Design review of the part built by this model. Coordinates are the model's own, in mm. A direction names the side the tool comes from. Give positions to 0.01 mm unless a question says otherwise; leave off trailing zeros. Write each loop counter-clockwise with the first axis right and the second up, starting at its lowest first coordinate (ties: lowest second). Pieces come first, ordered by that corner, then holes. Notation, with made-up numbers: (82.25, 9.5) -> (93.25, 9.5) arc R6 ccw to (93.25, 17.5) -> close; hole circle Ø3 at (8, 35.25). An arc over 180 degrees is marked (long way). Use CSV: the item, a comma, the result in double quotes.
```python
from build123d import *

# Parameters (mm, degrees)
BOSS_EXTRUDE2_DEPTH      = 3
BOSS_EXTRUDE2_DEPTH_BACK = 3
SKETCH2_W                = 50
SKETCH2_H                = 22
SKETCH2_W_2              = 22
SKETCH2_H_2              = 4
BOSS_EXTRUDE3_DEPTH      = 20
BOSS_EXTRUDE3_DEPTH_BACK = 20
SKETCH2_3_W              = 50
SKETCH2_3_H              = 3


with BuildPart() as part:
    # Sketch2 → Boss-Extrude2 (new, two sides: drawn at the far end of the back side and taken through both)
    with BuildSketch(Plane(origin=(0, 0, 0), x_dir=(0, 0, -1), z_dir=(1, 0, 0)).offset(-BOSS_EXTRUDE2_DEPTH_BACK)):
        with Locations((0, -1.5)):
            Rectangle(SKETCH2_W, SKETCH2_H)
        with Locations((0, -7.5)):
            Rectangle(SKETCH2_W_2, SKETCH2_H_2, mode=Mode.SUBTRACT)
    extrude(amount=BOSS_EXTRUDE2_DEPTH + BOSS_EXTRUDE2_DEPTH_BACK)

    # Sketch2<3> → Boss-Extrude3 (add, two sides: drawn at the far end of the back side and taken through both)
    with BuildSketch(Plane(origin=(0, 0, 0), x_dir=(0, 0, -1), z_dir=(1, 0, 0)).offset(-BOSS_EXTRUDE3_DEPTH_BACK)):
        with Locations((0, 11)):
            Rectangle(SKETCH2_3_W, SKETCH2_3_H)
    extrude(amount=BOSS_EXTRUDE3_DEPTH + BOSS_EXTRUDE3_DEPTH_BACK)


solid = part.part
```
(1) Tool access review of faces 5 (the face through (3, -1, 0)), 6 (the face through (0, -5.5, 0)), 7 (the face through (0, 12.5, 0)): name each direction out of +Z, -Z, +X, -X, +Y, -Y from which nothing blocks a thin tool from reaching the whole face with its end or side.
Established:
face 5,"+Z, -Z, +X, -Y"
face 6,"+X, -X"
face 7,"+Z, -Z, +X, -X, +Y"
(2) Take a section at D-D (x = 8). Write out the cut boundary in (y, z).
Established:
outline,"(9.5, -25) -> (12.5, -25) -> (12.5, 25) -> (9.5, 25) -> close"
(3) Take a section at B-B (x = -0.5). Write out the cut boundary in (y, z).
Established:
outline,"(-12.5, -25) -> (12.5, -25) -> (12.5, 25) -> (-12.5, 25) -> close; hole (-9.5, -11) -> (-5.5, -11) -> (-5.5, 11) -> (-9.5, 11) -> close"
(4) Clearance check with flat-ended pins moving along their axes: pin 1 (13.5 mm diameter, centred on x = -12.5, z = -6.5, fed in from -Y); pin 2 (13.5 mm diameter, centred on x = 8.5, z = -12, fed in from -Y); pin 3 (6 mm diameter, centred on y = -0.5, z = 9, fed in from +X); pin 4 (5 mm diameter, centred on y = -2.5, z = -8.5, fed in from -X). State where each tip first meets the part, or that it passes through.
Established:
pin 1,"stops at y = 9.5"
pin 2,"stops at y = -12.5"
pin 3,"stops at x = 3"
pin 4,"stops at x = -3"
(5) Take a section at C-C (z = 16). Write out the cut boundary in (x, y).
Established:
outline,"(-20, 9.5) -> (-3, 9.5) -> (-3, -12.5) -> (3, -12.5) -> (3, 9.5) -> (20, 9.5) -> (20, 12.5) -> (-20, 12.5) -> close"
(6) For line 1 along Y through (x, z) = (-17, -21.5); line 2 along X through (y, z) = (-1.5, 9); line 3 along Z through (x, y) = (0, -8), list the stretches that pass through material, from the lowest coordinate up. Write a range as [from, to].
Established:
line 1,"y = [9.5, 12.5]"
line 2,"x = [-3, 3]"
line 3,"z = [-25, -11], [11, 25]"
(7) Take a section at A-A (z = -1). Write out the cut boundary in (x, y), then the cut area to 3 significant figures.
Established:
outline,"(-20, 9.5) -> (-3, 9.5) -> (-3, -5.5) -> (3, -5.5) -> (3, 9.5) -> (20, 9.5) -> (20, 12.5) -> (-20, 12.5) -> close; (-3, -12.5) -> (3, -12.5) -> (3, -9.5) -> (-3, -9.5) -> close"
area,"228 mm2"
(8) Mouldability with a two-part tool opening along Y and no side actions: class faces 1 (the face through (0, -8, 11)), 2 (the face through (-12, 9.5, 0)), 3 (the face through (-3, -1, 0)), 4 (the face through (0, -9.5, 0)) as +Y half, -Y half, draft (parallel to the pull), parting line (faces both ways), or undercut.
Established:
face 1,"undercut"
face 2,"-Y half"
face 3,"draft"
face 4,"undercut"
